```python
from build123d import *

# Parameters (mm, degrees)
SKETCH_1_W          = 20
SKETCH_1_H          = 20
EXTRUDE_1_DEPTH     = 100
SKETCH_2_R          = 2
CUT_EXTRUDE_1_DEPTH = 20
SKETCH_3_R          = 2
CUT_EXTRUDE_2_DEPTH = 20
FILLET_1_R          = 1


with BuildPart() as part:
    # 草图1 → 凸台-拉伸1 (new body)
    with BuildSketch(Plane.XY):
        with Locations((10, 10)):
            Rectangle(SKETCH_1_W, SKETCH_1_H)
    extrude(amount=EXTRUDE_1_DEPTH)

    # 草图2 → 切除-拉伸1 (cut)
    with BuildSketch(Plane(origin=(20, 0, 0), x_dir=(0, 0, -1), z_dir=(1, 0, 0))):
        with Locations((-18, 10)):
            Circle(SKETCH_2_R)
        with Locations((-82, 10)):
            Circle(SKETCH_2_R)
    extrude(amount=-CUT_EXTRUDE_1_DEPTH, mode=Mode.SUBTRACT)

    # 草图3 → 切除-拉伸2 (cut)
    with BuildSketch(Plane.XZ):
        with Locations(Location((10, 90, 0), (0, 0, 270))):
            Circle(SKETCH_3_R)
    extrude(amount=-CUT_EXTRUDE_2_DEPTH, mode=Mode.SUBTRACT)

    # 圆角1
    fillet_1_edges = [part.edges().sort_by_distance(p)[0] for p in [
        (0, 20, 50),
        (20, 20, 50),
        (20, 0, 50),
        (0, 0, 50),
    ]]
    fillet(fillet_1_edges, radius=FILLET_1_R)


solid = part.part
```
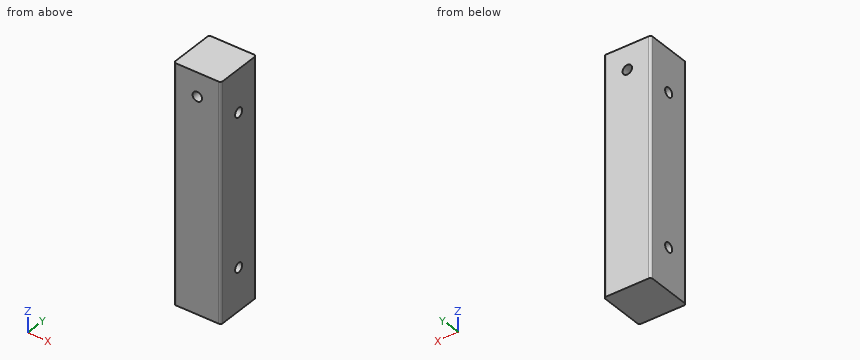
Can you work these out from the model? Positions are in its coordinate system, mm. Round coordinates to 2 decimals unless told otherwise and drop trailing zeros. Loops run counter-clockwise (first coordinate to the right, second up) from the corner with the lowest first, then second, coordinate; pieces in that order, holes last. Notation, with made-up numbers: M -37,32.25 L 13,32.25 A5 ccw 13,36.25 Z; hole C 30.5,87 d4. An arc over 180 degrees is marked long. Write item = value, one per line. Start each with the question number.
(1) Suppose I cut it at A-A on y = 10. Write out the boundary of the cut face in (x, z).
(2) I need wall thicknesses on line 1 along X through (y, z) = (12.5, 90); line 2 along Y through (x, z) = (8.25, 81). Which ranges of each line are inside material? Lowest first, please.
(3) Suppose I cut it at B-B on x = 10. Write out the boundary of the cut face in (y, z), plus the area to 3 significant figures.
(4) Suppose I cut it at C-C on z = 90. Write out the boundary of the cut face in (x, y).
Answer block:
q1.outline = M 0,0 L 20,0 L 20,16 L 0,16 Z; M 0,20 L 20,20 L 20,80 L 0,80 Z; M 0,84 L 20,84 L 20,100 L 0,100 Z; hole C 10,90 d4
q2.line_1 = 0 to 8, 12 to 20
q2.line_2 = 0 to 8.27, 11.73 to 20
q3.outline = M 0,0 L 20,0 L 20,88 L 0,88 Z; M 0,92 L 20,92 L 20,100 L 0,100 Z; hole C 10,18 d4; hole C 10,82 d4
q3.area = 1,890 mm²
q4.outline = M 0,1 A1 ccw 1,0 L 8,0 L 8,20 L 1,20 A1 ccw 0,19 Z; M 12,0 L 19,0 A1 ccw 20,1 L 20,19 A1 ccw 19,20 L 12,20 Z
